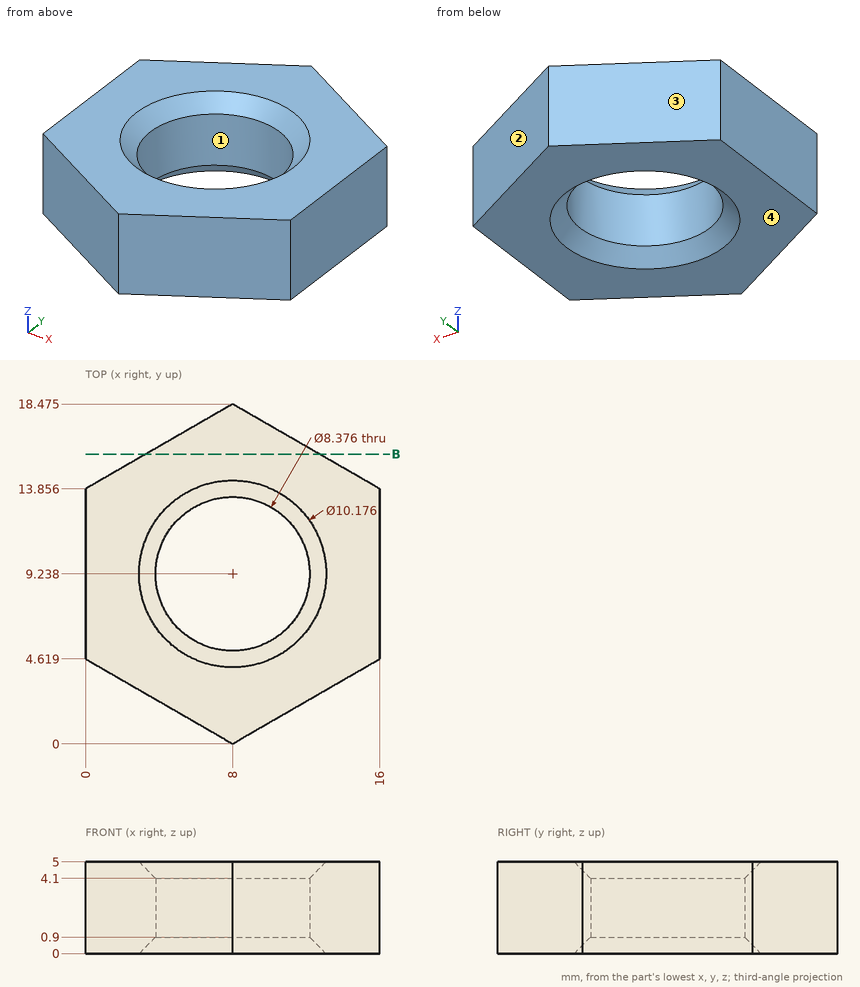
Study the drawing (mm; zero at the part's minimum x, y, z) and answer. Round coordinates to 2 decimals unless told otherwise and drop trailing zeros. Write each loop counter-clockwise with the first axis right and the second up, starting at its lowest first coordinate (ties: lowest second). Pieces come first, ordered by that corner, then holes.
1) Flat-ended cylindrical pins translate along their axes: P1, Ø1.5, axis at x = 2, z = 1.5, coming from the +Y side (1 decimal); P2, Ø3, axis at x = 6, z = 3.5, coming from the -Y side. Find the tip coordinate at first contact, or state that the pin passes through.
2) Consider probe 1 along X at (y, z) = (5.75, 2.9); probe 2 along X at (y, z) = (6.25, 2.9) (1 decimal); probe 3 along Y at (x, z) = (7, 3.6) (1 decimal). Determine where each line is inside the solid, lowest interval first.
3) Determine the mould class of the marked faces 1, 2, 3 and 4 for opening direction X: pulls with the +X half, pulls with the -X half, needs draft (parallel to the pull), parting line crosses it, or undercut.
4) A cutting plane is placed at B-B on y = 15.75. Determine the outline of the cut face in (x, z), and give its area (3 significant figures).
Entries:
1. P1: stops at y = 15.4
1. P2: stops at y = 0.29
2. probe 1: x = 0 to 5.68, 10.32 to 16
2. probe 2: x = 0 to 5.1, 10.9 to 16
2. probe 3: y = 0.6 to 5.2, 13.3 to 17.9
3. face 1: undercut
3. face 2: pulls with the +X half
3. face 3: pulls with the -X half
3. face 4: needs draft
4. outline: (3.28, 0) - (12.72, 0) - (12.72, 5) - (3.28, 5) - close
4. area: 47.2 mm2
